```python
from build123d import *

# Parameters (mm, degrees)
BOX003_W                 = 50
BOX003_H                 = 50
BOX003_DEPTH             = 10
BOX002_W                 = 10
BOX002_H                 = 110
BOX002_DEPTH             = 10
ARRAY001_X_COUNT         = 4
ARRAY001_X_PITCH         = 20
ARRAY001_PLACEMENT_ANGLE = 90
BOX001_W                 = 10
BOX001_H                 = 110
BOX001_DEPTH             = 10
ARRAY_X_COUNT            = 4
ARRAY_X_PITCH            = 20
BOX_W                    = 90
BOX_H                    = 90
BOX_DEPTH                = 150


with BuildPart() as cube003:
    # Box003 → Box003 (new body)
    with BuildSketch(Plane(origin=(20, 20, 140), x_dir=(1, 0, 0), z_dir=(0, 0, 1))):
        with Locations((25, 25)):
            Rectangle(BOX003_W, BOX003_H)
    extrude(amount=BOX003_DEPTH)


with BuildPart() as array001:
    # Box002 → Box002 (new body)
    with BuildSketch(Plane(origin=(10, -10, 140), x_dir=(1, 0, 0), z_dir=(0, 0, 1))):
        with Locations((5, 55)):
            Rectangle(BOX002_W, BOX002_H)
    extrude(amount=BOX002_DEPTH)

    # Array001 X: Array001 ×4


with BuildPart() as array001_1:
    add(array001.part)
    with Locations(*[(i * ARRAY001_X_PITCH, 0, 0) for i in range(1, ARRAY001_X_COUNT)]):
        add(array001.part)


with BuildPart() as array001_2:
    # Array001 placement: moved
    add(array001_1.part.moved(Location((90, 0, 0))).rotate(Axis((90, 0, 0), (0, 0, 1)), ARRAY001_PLACEMENT_ANGLE))


with BuildPart() as array:
    # Box001 → Box001 (new body)
    with BuildSketch(Plane(origin=(10, -10, 140), x_dir=(1, 0, 0), z_dir=(0, 0, 1))):
        with Locations((5, 55)):
            Rectangle(BOX001_W, BOX001_H)
    extrude(amount=BOX001_DEPTH)

    # Array X: Array ×4


with BuildPart() as array_1:
    add(array.part)
    with Locations(*[(i * ARRAY_X_PITCH, 0, 0) for i in range(1, ARRAY_X_COUNT)]):
        add(array.part)


with BuildPart() as cut002:
    # Box → Box (new body)
    with BuildSketch(Plane.XY):
        with Locations((45, 45)):
            Rectangle(BOX_W, BOX_H)
    extrude(amount=BOX_DEPTH)

    # Cut: cut Array
    add(array_1.part, mode=Mode.SUBTRACT)

    # Cut001: cut Array001
    add(array001_2.part, mode=Mode.SUBTRACT)

    # Cut002: cut Cube003
    add(cube003.part, mode=Mode.SUBTRACT)


solid = cut002.part
```
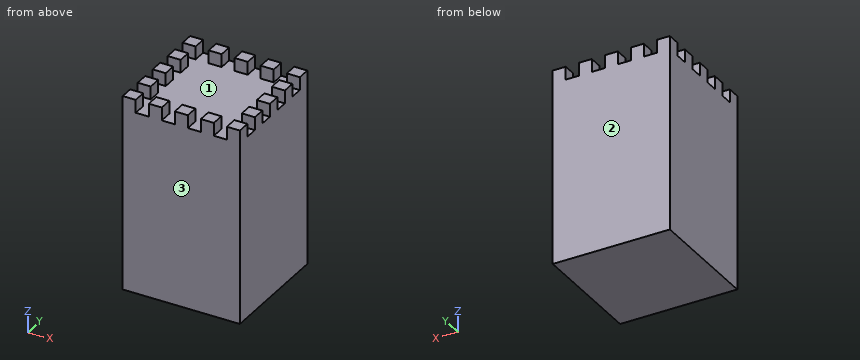
Source: CAD feature listing. Evaluate the final solid. Frame: model axes, mm. Face numbers are marked on the shaded views. Coordinates: 2 decimals unless noted, no trailing zeros. Loops run counter-clockwise (first coordinate to the right, second up) from the corner with the lowest first, then second, coordinate; pieces in that order, holes last. Notation, with made-up numbers: (60, 6.5) -> (98, 6.5) arc R23 ccw to (98, 39.5) -> close; hole circle Ø9 at (13.5, -23). An arc over 180 degrees is marked (long way). One line per item, written item: value. Start each with the question number.
Q1. Mould query, pull axis Y, two halves, no side actions, for the marked faces 1, 2 and 3. Classes: pulls with the +Y half, pulls with the -Y half, needs draft (parallel to the pull), parting line crosses it, or undercut.
Q2. Section query A-A, the plane y = 7. Return the cut outline in (x, z).
Q3. Section query C-C, the plane x = 28. Return the cut outline in (y, z).
Q4. Section query D-D, the plane y = 77.5. Return the cut outline in (x, z), and give its area (3 significant figures).
Q5. Line query: line 1 along Z through (x, y) = (66.5, 57). Output: solid intervals per line, ascending.
Q6. Contact query for flat-ended pins moving along their axis: P1, Ø6, axis at y = 23.5, z = 64, coming from the -X side; P2, Ø10, axis at x = 50, y = 22, coming from the +Z side. Output: stop coordinate, or through.
Results:
1. face 1: undercut
1. face 2: pulls with the +Y half
1. face 3: pulls with the -Y half
2. outline: (0, 0) -> (90, 0) -> (90, 150) -> (80, 150) -> (80, 140) -> (70, 140) -> (70, 150) -> (60, 150) -> (60, 140) -> (50, 140) -> (50, 150) -> (40, 150) -> (40, 140) -> (30, 140) -> (30, 150) -> (20, 150) -> (20, 140) -> (10, 140) -> (10, 150) -> (0, 150) -> close
3. outline: (0, 0) -> (90, 0) -> (90, 150) -> (80, 150) -> (80, 140) -> (10, 140) -> (10, 150) -> (0, 150) -> close
4. outline: (0, 0) -> (90, 0) -> (90, 140) -> (0, 140) -> close
4. area: 12,600 mm^2
5. line 1: 0 to 140
6. P1: x = 0
6. P2: z = 140
